Autodesk Inventor part; units mm, degrees
ref_plane "YZ Plane" through (0, 0, 0) normal (1, 0, 0) x (0, 1, 0)
ref_plane "XZ Plane" through (0, 0, 0) normal (0, 1, 0) x (-1, 0, 0)
ref_plane "XY Plane" through (0, 0, 0) normal (0, 0, 1) x (1, 0, 0)
sketch "Sketch1" plane through (0, 0, 0) normal (0, 0, 1) x (1, 0, 0)
  line L0 (-38.1, 50.8) -> (38.1, 50.8)
  line L1 (38.1, 50.8) -> (38.1, -50.8)
  line L2 (-38.1, -50.8) -> (-38.1, 50.8)
  circle A0 centre (0, 11.7) radius 11.1125
  line L3 (-38.1, -50.8) -> (0, -88.9)
  line L4 (0, -88.9) -> (38.1, -50.8)
  circle A1 centre (0, -50.8) radius 14.2875
  point P0 (0, 0)
  point P1 (-34.925, -47.625)
  point P2 (34.925, -47.625)
  point P3 (-34.925, 38.1)
  point P4 (34.925, 38.1)
  dimension "d0" = 76.2
  dimension "d1" = 38.1
  dimension "d2" = 101.6
  dimension "d3" = 50.8
  dimension "d4" = 101.6
  dimension "d5" = 38.1
  dimension "d6" = 38.1
  dimension "d7" = 28.575
  dimension "d8" = 38.1
  dimension "d9" = 38.1
  dimension "d10" = 22.225
  dimension "d11" = 38.1
  dimension "d13" = 3.175
  dimension "d14" = 12.7
  dimension "d15" = 3.175
  dimension "d16" = 3.175
  dimension "d17" = 3.175
  dimension "d18" = 3.175
  dimension "d31" = 3.175
  dimension "d32" = 12.7
  dimension "d88" = 62.5
extrude "Extrusion1" add sketch "Sketch1" against normal blind 6.35
fillet "Fillet1" radius 26.9494 1 edges at (0, -88.9, -3.175)
sketch "Sketch2" plane through (0, 0, 0) normal (0, 0, 1) x (1, 0, 0)
  line L0 (-38.1, 50.8) -> (38.1, 50.8)
  line L1 (-38.1, -50.8) -> (-38.1, 50.8)
  line L2 (38.1, -50.8) -> (19.0561, -69.8439)
  line L3 (38.1, 50.8) -> (38.1, -50.8)
  line L4 (-19.0561, -69.8439) -> (-38.1, -50.8)
  circle A0 centre (0, -50.8) radius 14.2875
  line L5 (-31.75, 44.45) -> (31.75, 44.45)
  line L6 (31.75, 44.45) -> (31.75, -48.1697)
  line L7 (-31.75, -48.1697) -> (-31.75, 44.45)
  line L8 (-31.75, -48.1697) -> (-20.4747, -59.445)
  line L9 (31.75, -48.1697) -> (20.4747, -59.445)
  arc A1 (20.4747, -59.445) -> (-20.4747, -59.445) centre (0, -50.8) ccw
  arc A2 (9.897, 26.0871) -> (-9.897, 26.0871) centre (0, 11.7) ccw
  arc A3 (14.3871, 1.803) -> (14.3871, 21.597) centre (0, 11.7) ccw
  arc A4 (-9.897, -2.6871) -> (9.897, -2.6871) centre (0, 11.7) ccw
  arc A5 (-14.3871, 21.597) -> (-14.3871, 1.803) centre (0, 11.7) ccw
  line L10 (0, 11.7) -> (-31.75, 43.45) construction
  line L11 (-31.75, 43.45) -> (0, 11.7) construction
  line L12 (0, 11.7) -> (31.75, 43.45) construction
  line L13 (0, 11.7) -> (-31.75, -20.05) construction
  line L14 (0, 11.7) -> (31.75, -20.05) construction
  line L15 (-31.75, 38.9599) -> (-14.3871, 21.597) construction
  line L16 (-14.3871, 21.597) -> (-31.75, 38.9599)
  line L17 (-28.2599, 44.45) -> (-9.897, 26.0871)
  line L18 (28.2599, 44.45) -> (9.897, 26.0871)
  line L19 (31.75, 38.9599) -> (14.3871, 21.597)
  line L20 (31.75, -15.5599) -> (14.3871, 1.803)
  line L21 (14.3871, 1.803) -> (31.75, -15.5599)
  line L22 (31.75, -24.5401) -> (9.897, -2.6871)
  line L23 (-31.75, -24.5401) -> (-9.897, -2.6871)
  line L24 (-31.75, -15.5599) -> (-14.3871, 1.803)
  line L25 (-31.75, -20.05) -> (0, -50.8) construction
  line L26 (0, -50.8) -> (31.75, -20.05) construction
  line L27 (-18.0398, -37.8186) -> (-31.75, -24.5401)
  line L28 (31.75, -24.5401) -> (18.396, -38.3285)
  line L29 (27.2599, -20.05) -> (14.1094, -33.6281)
  line L30 (-27.2593, -20.0494) -> (-13.6325, -33.247)
  point P0 (38.1, -47.625)
  point P1 (38.1, 41.275)
  point P2 (25.4, 50.8)
  point P3 (-25.4, 50.8)
  point P4 (-38.1, 41.275)
  point P5 (-38.1, -47.625)
  point P6 (-34.925, 38.1)
  point P7 (-34.925, -47.625)
  point P8 (34.925, 38.1)
  point P9 (34.925, -47.625)
  dimension "d92" = 12.7
  dimension "d93" = 3.175
  dimension "d96" = 85.725
  dimension "d99" = 69.85
  dimension "d106" = 6.35
  dimension "d107" = 6.35
  dimension "d108" = 6.35
  dimension "d109" = 6.35
  dimension "d110" = 6.35
  dimension "d111" = 22.225
  dimension "d112" = 17.4625
  dimension "d113" = 6.35
  dimension "d114" = 3.175
  dimension "d115" = 6.35
  dimension "d116" = 3.175
  dimension "d117" = 6.35
  dimension "d118" = 3.175
  dimension "d119" = 6.35
  dimension "d120" = 3.175
  dimension "d121" = 6.35
  dimension "d122" = 6.3492
hole "Hole3" at (-34.925, -47.625, 0) at (34.925, -47.625, 0) at (-34.925, 38.1, 0) at (34.925, 38.1, 0) direction (0, 0, -1) diameter 3.175 end through all countersink diameter 6.35 countersink angle 82
sketch "Sketch3" plane through (-38.1, 50.8, 0) normal (0, 1, 0) x (1, 0, 0)
  line L0 (0, 0) -> (0, 6.35)
  line L1 (0, 0) -> (76.2, 0)
  line L2 (76.2, 0) -> (76.2, 6.35)
  point P0 (38.1, 0)
  point P1 (3.175, 3.175)
  point P2 (73.025, 3.175)
  dimension "d77" = 3.175
  dimension "d78" = 3.175
  dimension "d79" = 3.175
hole "Hole4" at (-34.925, 50.8, -3.175) at (34.925, 50.8, -3.175) direction (0, -1, 0) diameter 3.175 depth 9.525 tip angle 118
extrude "Extrusion4" cut sketch "Sketch2" against normal blind 25.4 contours L5 L18 A2 L17 | L16 A5 L24 L7 | L27 A1 L8 L7 | L6 L20 A3 L19 | L23 A4 L22 L29 A1 L30 | L6 L9 A1 L28
fillet "Fillet4" radius 3.175 26 edges at (-28.2599, 44.45, -3.175) (-9.897, 26.0871, -3.175) (28.2599, 44.45, -3.175) (9.897, 26.0871, -3.175) (14.3871, 21.597, -3.175) (-14.3871, 1.803, -3.175) (14.3871, 1.803, -3.175) (31.75, 38.9599, -3.175) (-14.3871, 21.597, -3.175) (-31.75, 38.9599, -3.175) (-31.75, -15.5599, -3.175) (31.75, -15.5599, -3.175) (9.897, -2.6871, -3.175) (-9.897, -2.6871, -3.175) (-27.2593, -20.0494, -3.175) (27.2599, -20.05, -3.175) (14.1094, -33.6281, -3.175) (-13.6325, -33.247, -3.175) (-31.75, -24.5401, -3.175) (-18.0398, -37.8186, -3.175) (-31.75, -48.1697, -3.175) (-20.4747, -59.445, -3.175) (20.4747, -59.445, -3.175) (31.75, -48.1697, -3.175) (31.75, -24.5401, -3.175) (18.396, -38.3285, -3.175)
equation "\"d108\" = d106"
equation "\"d109\" = d108"
equation "\"d110\" = d109"
properties part number "Lower box side plate"
Read the model definition and answer for the solid it produces. Units are mm, in the model's axes. A direction names the side the tool comes from. Round coordinates to 2 decimals unless told otherwise and drop trailing zeros. Loops run counter-clockwise (first coordinate to the right, second up) from the corner with the lowest first, then second, coordinate; pieces in that order, holes last. Notation, with made-up numbers: (29.5, 37.25) -> (72.5, 37.25) arc R21 ccw to (72.5, 73.25) -> close; hole circle Ø7 at (67, -34.75). An arc over 180 degrees is marked (long way). One line per item, written item: value.
1) The mould has two halves that part along Z. Classify faces 1 (the face through (-35.093, 40.487, -3.394)), 2 (the face through (-1, 50.8, -3)), 3 (the face through (8, 2, -6.35)): pulls with the +Z half, pulls with the -Z half, needs draft (parallel to the pull), parting line crosses it, or undercut.
Answer list:
face 1: undercut
face 2: needs draft
face 3: pulls with the -Z half
2) For faces 4 (the face through (36.475, 45.971, -3.519)), 5 (the face through (-29.25, -50.67, -3.13)), 6 (the face through (8, 2, 0)), determine the directions among +Z, -Z, +X, -X, +Y, -Y from which every point of the face is accessible in a straight line to the end or side of a thin tool.
Answer list:
face 4: +Y
face 5: +Z, -Z
face 6: +Z, +X, -X, +Y, -Y
3) A cutting plane is placed at A-A (x = 0). Determine the outline of the cut face in (y, z), and give its area (3 significant figures).
Answer list:
outline: (-77.74, -6.35) -> (-65.09, -6.35) -> (-65.09, 0) -> (-77.74, 0) -> close; (-36.51, -6.35) -> (-28.58, -6.35) -> (-28.58, 0) -> (-36.51, 0) -> close; (-5.76, -6.35) -> (0.59, -6.35) -> (0.59, 0) -> (-5.76, 0) -> close; (22.81, -6.35) -> (29.16, -6.35) -> (29.16, 0) -> (22.81, 0) -> close; (44.45, -6.35) -> (50.8, -6.35) -> (50.8, 0) -> (44.45, 0) -> close
area: 252 mm²
4) Consider L1, parallel to Y at x = 31.5, z = -4.5; L2, parallel to X at y = 10, z = -5.5; L3, parallel to Y at x = -28, z = -4.5. Determine where each line is inside the solid, lowest interval first. Write a range as [from, to].
Answer list:
L1: y = [-57.4, -48.09], [-31.15, -9.13], [32.53, 50.8]
L2: x = [-38.1, -31.75], [-17.38, -10.98], [10.98, 17.38], [31.75, 38.1]
L3: y = [-60.9, -51.92], [-28.91, -11.02], [34.42, 50.8]
5) A cutting plane is placed at B-B (y = 11.7). Determine the outline of the cut face in (x, z).
Answer list:
outline: (-38.1, -6.35) -> (-31.75, -6.35) -> (-31.75, 0) -> (-38.1, 0) -> close; (-17.46, -6.35) -> (-11.11, -6.35) -> (-11.11, 0) -> (-17.46, 0) -> close; (11.11, -6.35) -> (17.46, -6.35) -> (17.46, 0) -> (11.11, 0) -> close; (31.75, -6.35) -> (38.1, -6.35) -> (38.1, 0) -> (31.75, 0) -> close
6) A cutting plane is placed at C-C (y = -27). Determine the outline of the cut face in (x, z), and give its area (3 significant figures).
Answer list:
outline: (-38.1, -6.35) -> (-20.08, -6.35) -> (-20.08, 0) -> (-38.1, 0) -> close; (20.53, -6.35) -> (38.1, -6.35) -> (38.1, 0) -> (20.53, 0) -> close
area: 226 mm²
7) Flat-ended cylindrical pins translate along their axes: P1, Ø2.5, axis at x = 34.925, z = -3.175, coming from the +Y side; P2, Ø1.9, axis at x = -34.925, z = -3.175, coming from the +Y side. Find the tip coordinate at first contact, or state that the pin passes through.
Answer list:
P1: stops at y = 41.07
P2: stops at y = 40.89
